from build123d import *

# Parameters (mm, degrees)
EXTRUDE1_DEPTH = 0.7
EXTRUDE2_DEPTH = 1
DRAFT1_ANGLE   = 45


with BuildPart() as part:
    # Sketch1 → Extrude1 (new body)
    with BuildSketch(Plane.XY):
        with BuildLine():
            Line((19.155576725, 24.033479545), (19.153057259, 24.033479546))
            ThreePointArc((19.153057259, 24.033479546), (18.688120429, 23.858493389), (18.453932737, 23.42038092))
            Line((18.453932737, 23.42038092), (18.453932737, 10.52156184))
            ThreePointArc((18.453932737, 10.52156184), (23.954511515, 11.07234739), (29.455090293, 10.52156184))
            Line((29.455090293, 10.52156184), (29.455090293, 14.303453829))
            Line((29.455090293, 14.303453829), (28.809678981, 15.087349513))
            Line((28.809678981, 15.087349513), (28.809678981, 16.030799168))
            Line((28.809678981, 16.030799168), (29.465965334, 16.405404217))
            Line((29.465965334, 16.405404217), (29.465965334, 17.856041137))
            Line((29.465965334, 17.856041137), (28.185089103, 19.147527308))
            Line((28.185089103, 19.147527308), (28.185089103, 23.42038092))
            ThreePointArc((28.185089103, 23.42038092), (27.949953539, 23.859323131), (27.483445115, 24.033475046))
            Line((27.483445115, 24.033475046), (19.155576725, 24.033479545))
        make_face()
        with BuildLine():
            Line((19.382079549, 9.033491555), (28.526943481, 9.033491554))
            ThreePointArc((28.526943481, 9.033491554), (29.202633724, 9.645535961), (29.455090293, 10.52156184))
            ThreePointArc((29.455090293, 10.52156184), (23.954511515, 11.07234739), (18.453932737, 10.52156184))
            ThreePointArc((18.453932737, 10.52156184), (18.702527644, 9.643127345), (19.382079549, 9.033491555))
        make_face()
    extrude(amount=EXTRUDE1_DEPTH)

    # Sketch2 → Extrude2 (add)
    with BuildSketch(Plane.XY):
        with BuildLine():
            Line((19.382079549, 9.033491555), (28.526943481, 9.033491554))
            ThreePointArc((28.526943481, 9.033491554), (29.202633724, 9.645535961), (29.455090293, 10.52156184))
            ThreePointArc((29.455090293, 10.52156184), (23.954511515, 11.072347393), (18.453932737, 10.52156184))
            ThreePointArc((18.453932737, 10.52156184), (18.702527644, 9.643127345), (19.382079549, 9.033491555))
        make_face()
    extrude(amount=EXTRUDE2_DEPTH)

    # Draft1
    draft1_faces = [part.faces().sort_by_distance(p)[0] for p in [
        (23.954511515, 11.072347393, 0.85),
    ]]
    draft(draft1_faces, Plane(origin=(23.959933723, 1.918279908, 0.7), x_dir=(1, 0, 0), z_dir=(0, 0, 1)), DRAFT1_ANGLE)


solid = part.part
Design review of the part built by this model. Coordinates are the model's own, in mm. Give positions to 0.01 mm unless a question says otherwise; leave off trailing zeros. Loops run counter-clockwise (first coordinate to the right, second up) from the corner with the lowest first, then second, coordinate; pieces in that order, holes last. Notation, with made-up numbers: M -21.75,12.5 L 6.25,12.5 A19 cw 6.25,17.5 Z; hole C -24.75,86 d5. An arc over 180 degrees is marked long. Answer as a JSON object with one key per item and string values.
Item 1: We need section B-B (y = 19.5). State the section outline as (x, z) points, and give its area (3 significant figures).
Output values:
{"outline": "M 18.45,0 L 28.19,0 L 28.19,0.7 L 18.45,0.7 Z", "area": "6.81 mm2"}
Item 2: For P1, Ø4, axis at x = 26.5, y = 14.5, coming from the +Z side; P2, Ø0.6, axis at y = 21, z = 0.5, coming from the +X side, all flat-tipped, find the tip position at first contact; note any pin that passes through.
Output values:
{"P1": "stops at z = 0.7", "P2": "stops at x = 28.19"}
Item 3: Wall thickness on line 1 along Z through (x, y) = (26, 17.5); line 2 along Y through (x, z) = (29, 0.55); line 3 along X through (y, z) = (11.5, 0.55): over which ranges is each line inside the solid? List them lowest first.
Output values:
{"line 1": "z = 0 to 0.7", "line 2": "y = 9.38 to 14.86, 16.14 to 18.33", "line 3": "x = 18.45 to 29.46"}
Item 4: We need section C-C (y = 15.25). State the section outline as (x, z) points.
Output values:
{"outline": "M 18.45,0 L 28.81,0 L 28.81,0.7 L 18.45,0.7 Z"}
